Input: part model. Units: mm. Frame: model coordinates. A direction names the side the tool comes from. Give positions to 0.01 mm unless a question says otherwise; leave off trailing zeros. Loops run counter-clockwise (first coordinate to the right, second up) from the corner with the lowest first, then second, coordinate; pieces in that order, holes last. Notation, with made-up numbers: M 13,49.25 L 46,49.25 A25 cw 46,73.25 Z; hole C 26.5,15.5 d11. An arc over 180 degrees is marked long. Return JSON: item names as keys, results as strings. Group by question number.
```python
from build123d import *

# Parameters (mm, degrees)
SKETCH1_W           = 55.245
SKETCH1_H           = 54.991
BOSS_EXTRUDE1_DEPTH = 12.7
SKETCH2_W           = 53.645
SKETCH2_H           = 53.391
CUT_EXTRUDE1_DEPTH  = 11.9
CUT_EXTRUDE2_DEPTH  = 11.9


with BuildPart() as part:
    # Sketch1 → Boss-Extrude1 (new body)
    with BuildSketch(Plane(origin=(0, 0, 0), x_dir=(1, 0, 0), z_dir=(0, 1, 0))):
        with Locations((108.93085592, -3.252731307)):
            Rectangle(SKETCH1_W, SKETCH1_H)
    extrude(amount=BOSS_EXTRUDE1_DEPTH)

    # Sketch2 → Cut-Extrude1 (cut)
    with BuildSketch(Plane(origin=(0, 12.7, 0), x_dir=(1, 0, 0), z_dir=(0, 1, 0))):
        with Locations((108.93085592, -3.252731307)):
            Rectangle(SKETCH2_W, SKETCH2_H)
    extrude(amount=-CUT_EXTRUDE1_DEPTH, mode=Mode.SUBTRACT)

    # Sketch3 → Cut-Extrude2 (cut)
    with BuildSketch(Plane(origin=(0, 0.8, 0), x_dir=(1, 0, 0), z_dir=(0, 1, 0))):
        Polygon((88.811093554, 3.029967001), (104.660142286, 1.203676379), (104.521442297, 0), (88.672393566, 1.826290622), align=None)
        Polygon((94.647979747, 12.248126215), (107.460513263, 2.741987776), (106.73855736, 1.768923448), (93.926023844, 11.275061887), align=None)
        Polygon((104.311951076, 17.312843174), (110.654861369, 2.674019035), (109.543097052, 2.19229856), (103.20018676, 16.831122698), align=None)
        Polygon((115.213554228, 16.867031059), (113.387263606, 1.017982327), (112.183587227, 1.156682316), (114.009877849, 17.005731048), align=None)
        Polygon((124.431713442, 11.030144866), (114.925575003, -1.78238865), (113.952510675, -1.060432747), (123.458649114, 11.752100769), align=None)
        Polygon((129.496430401, 1.366173537), (114.857606263, -4.976736755), (114.375885787, -3.864972439), (129.014709925, 2.477937854), align=None)
        Polygon((129.050618286, -9.535429615), (113.201569555, -7.709138993), (113.340269543, -6.505462614), (129.189318275, -8.331753236), align=None)
        Polygon((123.213732093, -18.753588829), (110.401198577, -9.24745039), (111.12315448, -8.274386062), (123.935687997, -17.780524501), align=None)
        Polygon((113.549760764, -23.818305788), (107.206850472, -9.17948165), (108.318614788, -8.697761174), (114.661525081, -23.336585312), align=None)
        Polygon((102.648157613, -23.372493673), (104.474448234, -7.523444941), (105.678124613, -7.66214493), (103.851833991, -23.511193662), align=None)
        Polygon((93.429998399, -17.53560748), (102.936136838, -4.723073964), (103.909201165, -5.445029867), (94.403062726, -18.257563383), align=None)
        Polygon((88.365281439, -7.871636151), (103.004105578, -1.528725859), (103.485826053, -2.640490175), (88.847001915, -8.983400468), align=None)
    extrude(amount=-CUT_EXTRUDE2_DEPTH, mode=Mode.SUBTRACT)


solid = part.part
```
Item 1: Material intervals for line 1 (Z direction, x = 103, y = 3); line 2 (X direction, y = 12, z = 14); line 3 (Y direction, x = 101, z = 4), sorted ascending. Write a range as from..to.
Item 2: Section C-C, the plane z = -19.5. Return loops of the section in (x, y).
Item 3: First-contact query: pin 1 Ø1 at (x, z) = (105, -11.5) entering from -Y. Flat tip, straight axial feed; report the tip coordinate or a pass-through.
Item 4: Section B-B, the plane x = 95.5. Return loops of the section in (y, z), then the cut area to 3 significant figures.
Item 5: Reachability of faces 1 (the face through (100.422, 0.406, -6.455)), 2 (the face through (109, 0.8, 3)) from +Z, -Z, +X, -X, +Y, -Y: full face, straight path, thin tool, end or side. Return the list, or none.
Item 6: Section A-A, the plane y = 9.75. Return loops of the section in (x, z), then the cut area to 3 significant figures.
Item 7: Section D-D, the plane x = 85. Return loops of the section in (y, z).
Answer below:
{
 "1": {"line 1": "-24.24..-23.44, 29.95..30.75", "line 2": "81.31..82.11, 135.75..136.55", "line 3": "0..0.8"},
 "2": {"outline": "M 81.31,0 L 136.55,0 L 136.55,12.7 L 135.75,12.7 L 135.75,0.8 L 82.11,0.8 L 82.11,12.7 L 81.31,12.7 Z"},
 "3": {"pin 1": "y = 0"},
 "4": {"outline": "M 0,-24.24 L 12.7,-24.24 L 12.7,-23.44 L 0.8,-23.44 L 0.8,-11.62 L 0,-11.62 Z; M 0,-10.11 L 0.8,-10.11 L 0.8,-2.26 L 0,-2.26 Z; M 0,-1.04 L 0.8,-1.04 L 0.8,4.78 L 0,4.78 Z; M 0,6.1 L 0.8,6.1 L 0.8,14.75 L 0,14.75 Z; M 0,16.78 L 0.8,16.78 L 0.8,29.95 L 12.7,29.95 L 12.7,30.75 L 0,30.75 Z", "area": "58.2 mm^2"},
 "5": {"face 1": "+Y, -Y", "face 2": "+Y"},
 "6": {"outline": "M 81.31,-24.24 L 136.55,-24.24 L 136.55,30.75 L 81.31,30.75 Z; hole M 82.11,-23.44 L 135.75,-23.44 L 135.75,29.95 L 82.11,29.95 Z", "area": "174 mm^2"},
 "7": {"outline": "M 0,-24.24 L 12.7,-24.24 L 12.7,-23.44 L 0.8,-23.44 L 0.8,29.95 L 12.7,29.95 L 12.7,30.75 L 0,30.75 Z"}
}
